Here's the drawing with two shaded views (mm, measured from the low corner). I have some questions. A direction names the side the tool comes from. Coordinates: 2 decimals unless noted, no trailing zeros. Order: outer loops, then holes, each group sorted by start corner. A loop starts at its lowest first (then second) coordinate and runs counter-clockwise, first axis right, second up. Notation, with made-up numbers: (74.25, -23.5) - (85.25, -23.5) arc R29 cw to (85.25, 4.5) - close; hole circle Ø10 at (57, -1). An arc over 180 degrees is marked (long way). Answer as a JSON object with one key per item and string values. Group by question number.
(1) Imagine slicing it at D-D, the plane x = 36. Write out the boundary of the cut face in (y, z).
(2) Imagine slicing it at C-C, the plane z = 4.5. Write out the boundary of the cut face in (x, y), and give its area (3 significant figures).
(3) Will these pins go through, and if not, where does the flat tip stop? P1, Ø12, axis at y = 28, z = 24.5, coming from the +X side; P2, Ø1, axis at y = 7.5, z = 15.5, coming from the -X side; P3, Ø1, axis at y = 13.5, z = 15, coming from the -X side.
(4) Please list where these lines run through material, in increasing order: probe 1 along X at (y, z) = (63, 20); probe 2 along Y at (x, z) = (15, 7); probe 3 along X at (y, z) = (63.95, 8).
(5) We'd pull the mould along Y, two halves only. Please class the marked faces 1, 2 and 3: pulls with the +Y half, pulls with the -Y half, needs draft (parallel to the pull), parting line crosses it, or undercut.
(6) Imagine slicing it at B-B, the plane z = 21. Write out the boundary of the cut face in (x, y), and give its area (3 significant figures).
(7) Which directions (+Z, -Z, +X, -X, +Y, -Y) give clear straight access to the entire face, cutting with the end or side of a thin tool? Please do the marked faces 4 and 5.
(8) Imagine slicing it at A-A, the plane x = 20. Write out the boundary of the cut face in (y, z).
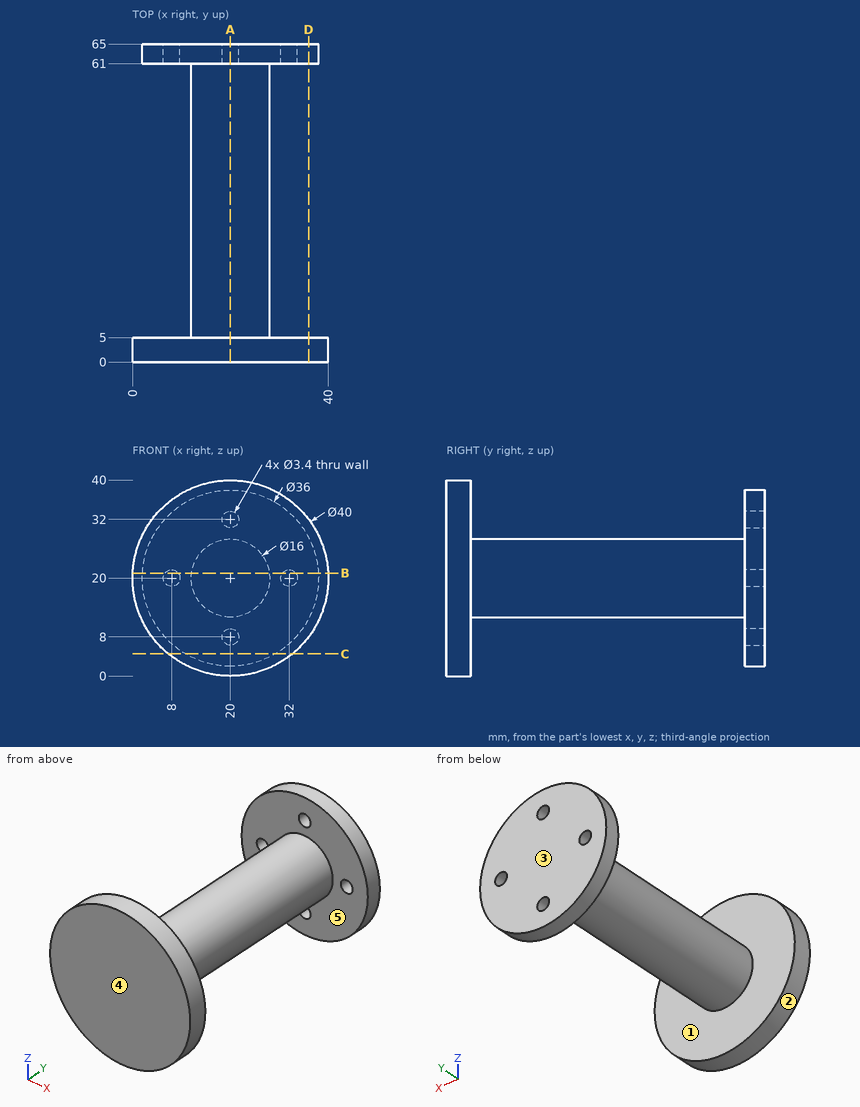
Result set:
{
 "1": {"outline": "(0, 8) - (5, 8) - (5, 32) - (0, 32) - close; (61, 11.75) - (65, 11.75) - (65, 28.25) - (61, 28.25) - close"},
 "2": {"outline": "(7.36, 0) - (32.64, 0) - (32.64, 5) - (7.36, 5) - close; (10.85, 61) - (29.15, 61) - (29.15, 65) - (10.85, 65) - close", "area": "200 mm^2"},
 "3": {"P1": "stops at x = 28", "P2": "stops at x = 13.07", "P3": "stops at x = 13.39"},
 "4": {"probe 1": "x = 2 to 6.3, 9.7 to 30.3, 33.7 to 38", "probe 2": "y = 0 to 5, 61 to 65", "probe 3": "x = 6.58 to 18.3, 21.7 to 33.42"},
 "5": {"face 1": "undercut", "face 2": "needs draft", "face 3": "pulls with the +Y half"},
 "6": {"outline": "(0.03, 0) - (39.97, 0) - (39.97, 5) - (27.94, 5) - (27.94, 61) - (30.63, 61) - (30.63, 65) - (9.37, 65) - (9.37, 61) - (12.06, 61) - (12.06, 5) - (0.03, 5) - close; (2.03, 61) - (6.63, 61) - (6.63, 65) - (2.03, 65) - close; (33.37, 61) - (37.97, 61) - (37.97, 65) - (33.37, 65) - close", "area": "1,210 mm^2"},
 "7": {"face 4": "+Z, -Z, +X, -X, -Y", "face 5": "none"},
 "8": {"outline": "(0, 0) - (5, 0) - (5, 12) - (61, 12) - (61, 9.7) - (65, 9.7) - (65, 30.3) - (61, 30.3) - (61, 28) - (5, 28) - (5, 40) - (0, 40) - close; (61, 2) - (65, 2) - (65, 6.3) - (61, 6.3) - close; (61, 33.7) - (65, 33.7) - (65, 38) - (61, 38) - close"}
}
